Autodesk Fusion 360 part; units mm, degrees
sketch "Sketch1" plane through (0, 0, 0) normal (0, 0, 1) x (1, 0, 0) in component "Airfoil structure"
  spline S0 degree 5 poles (152.8506, 9.5306) (153.6754, 9.3537) (155.1958, 9.0287) (157.0885, 8.6275) (158.936, 8.2427) (160.6637, 7.8881) (162.4454, 7.5151) (164.8303, 6.998) (168.0437, 6.2836) (171.9513, 5.3996) (176.2204, 4.4167) (180.4193, 3.4264) (184.1364, 2.5129) (187.0894, 1.7283) (189.2467, 1.0645) (190.9412, 0.4268) (192.3181, -0.1665) (193.5665, -0.7111) (194.5238, -1.126) (195.0337, -1.3464) knots 0 0 0 0 0 0 0.066667 0.133333 0.2 0.266667 0.333333 0.4 0.466667 0.533333 0.6 0.666667 0.733333 0.8 0.866667 0.933333 1 1 1 1 1 1
  line L0 (148.4907, 10.4656) -> (157.2105, 8.5955)
  line L1 (191.9852, -0.0289) -> (198.0822, -2.6639)
  circle A0 centre (33.1388, 9.1296) radius 4.765
  circle A1 centre (116.1615, 7.0362) radius 3.175
  spline S1 degree 5 poles (-3.081, -1.3464) (-3.6016, -1.2536) (-4.5414, -1.0763) (-5.6463, -0.8353) (-6.5938, -0.5669) (-7.329, -0.2953) (-8.0513, 0.0089) (-9.0194, 0.5707) (-10.0683, 1.7874) (-10.9642, 3.2518) (-11.5103, 4.4866) (-11.5777, 5.0951) (-11.407, 5.643) (-11.0112, 6.6067) (-10.1307, 7.993) (-8.6022, 9.6431) (-6.4035, 11.272) (-4.1965, 12.5715) (-2.7349, 13.4061) (-1.8316, 13.8946) (-1.0216, 14.2664) (0.0955, 14.6934) (1.459, 15.1916) (2.6392, 15.6173) (3.2971, 15.8534) knots 0 0 0 0 0 0 0.05 0.1 0.15 0.2 0.25 0.3 0.35 0.4 0.45 0.5 0.55 0.6 0.65 0.7 0.75 0.8 0.85 0.9 0.95 1 1 1 1 1 1
  line L2 (0.5703, -1.9971) -> (-6.7323, -0.6957)
  line L3 (-0.0118, 14.6656) -> (6.606, 17.0412)
  line L4 (-8.4792, 9.8153) -> (-3.9569, 12.8132)
  line L5 (-11.5034, 4.2257) -> (-11.5345, 5.6935)
  line L6 (-7.2174, -0.5359) -> (-9.7443, 1.1286)
  spline S2 degree 5 poles (93.5688, 19.3646) (93.8188, 19.3387) (94.2829, 19.2905) (94.8714, 19.229) (95.4658, 19.1659) (96.0263, 19.1049) (96.567, 19.0445) (97.2368, 18.9678) (98.1315, 18.8622) (99.313, 18.7173) (100.8214, 18.5245) (102.3118, 18.3263) (103.5973, 18.1504) (104.53, 18.0207) (105.0153, 17.9528) knots 0 0 0 0 0 0 0.1 0.2 0.3 0.4 0.5 0.6 0.7 0.8 0.9 1 1 1 1 1 1
  line L7 (92.266, 19.4996) -> (94.8715, 19.2297)
  line L8 (103.6448, 18.1447) -> (106.3858, 17.761)
  spline S3 degree 5 poles (6.5765, 16.943) (6.9079, 17.0449) (7.5374, 17.2364) (8.3817, 17.4868) (9.3156, 17.7508) (10.2084, 17.9865) (10.8922, 18.156) (11.4504, 18.29) (11.9864, 18.4184) (12.6265, 18.5675) (13.504, 18.76) (14.4962, 18.9637) (15.447, 19.1503) (16.1786, 19.2906) (16.5688, 19.3646) knots 0 0 0 0 0 0 0.1 0.2 0.3 0.4 0.5 0.6 0.7 0.8 0.9 1 1 1 1 1 1
  line L9 (5.4107, 16.5846) -> (7.7424, 17.3015)
  line L10 (15.2328, 19.111) -> (17.9048, 19.6183)
  line L11 (152.4045, 9.626) -> (152.8506, 9.5306)
  line L12 (107.9851, 17.5282) -> (108.4359, 17.4637)
  line L13 (6.1441, 16.7993) -> (6.5765, 16.943)
  line L14 (128.8588, -1.3464) -> (132.3138, -1.3464)
  line L15 (149.471, 10.2539) -> (148.8431, 7.3203)
  line L16 (148.8431, 7.3203) -> (151.7767, 6.6925)
  line L17 (151.7767, 6.6925) -> (152.4045, 9.626)
  line L18 (3.2971, 15.8534) -> (4.243, 13.0064)
  line L19 (4.243, 13.0064) -> (7.09, 13.9524)
  line L20 (7.09, 13.9524) -> (6.1441, 16.7993)
  line L21 (160.8934, -1.3464) -> (160.8934, 1.6536)
  line L22 (160.8934, 1.6536) -> (163.8934, 1.6536)
  line L23 (163.8934, 1.6536) -> (163.8934, -1.3464)
  line L24 (132.3138, -1.3464) -> (160.8934, -1.3464)
  line L25 (163.8934, -1.3464) -> (195.0337, -1.3464)
  line L26 (3.4513, -1.3464) -> (3.4513, 1.6536)
  line L27 (3.4513, 1.6536) -> (6.4513, 1.6536)
  line L28 (6.4513, 1.6536) -> (6.4513, -1.3464)
  line L29 (-3.081, -1.3464) -> (3.4513, -1.3464)
  line L30 (105.0153, 17.9528) -> (107.9851, 17.5282)
  line L31 (19.5688, 19.3646) -> (19.5688, 16.3646)
  line L32 (19.5688, 16.3646) -> (16.5688, 16.3646)
  line L33 (16.5688, 16.3646) -> (16.5688, 19.3646)
  line L34 (90.5688, 19.3646) -> (90.5688, 16.3646)
  line L35 (90.5688, 16.3646) -> (93.5688, 16.3646)
  line L36 (93.5688, 16.3646) -> (93.5688, 19.3646)
  line L37 (113.7881, 13.5683) -> (110.8279, 14.0557)
  line L38 (110.8279, 14.0557) -> (111.3153, 17.0159)
  line L39 (113.7881, 13.5683) -> (114.2755, 16.5285)
  spline S4 degree 5 poles (108.4359, 17.4637) (108.6467, 17.433) (108.9931, 17.3831) (109.2865, 17.3426) (109.4547, 17.3194) (110.0313, 17.2264) (110.7239, 17.113) (111.2088, 17.0334) (111.3153, 17.0159) knots 0 0 0 0 0 0 0.066667 0.133333 0.2 0.217791 0.217791 0.217791 0.217791 0.217791 0.217791
  line L40 (107.9387, 17.5361) -> (108.933, 17.3913)
  line L41 (110.8712, 17.0888) -> (111.7595, 16.9429)
  spline S5 degree 5 poles (114.2755, 16.5285) (114.9096, 16.424) (116.2698, 16.2) (118.5862, 15.8186) (122.1455, 15.233) (126.9408, 14.4438) (131.5558, 13.6821) (135.521, 13.0215) (138.5596, 12.5011) (140.775, 12.0942) (142.7661, 11.6889) (144.7964, 11.2532) (146.8777, 10.807) (148.5577, 10.4484) (149.471, 10.2539) knots 0 0 0 0 0 0 0.1 0.2 0.3 0.4 0.5 0.6 0.7 0.8 0.9 1 1 1 1 1 1
  line L42 (111.4536, 16.9934) -> (117.0973, 16.0636)
  line L43 (143.5745, 11.5101) -> (155.3674, 8.9976)
  line L44 (56.6502, 19.3646) -> (56.6502, 16.3646)
  line L45 (56.6502, 16.3646) -> (53.6502, 16.3646)
  line L46 (53.6502, 16.3646) -> (53.6502, 19.3646)
  line L47 (19.5688, 19.3646) -> (53.6502, 19.3646)
  line L48 (56.6502, 19.3646) -> (90.5688, 19.3646)
  line L49 (68.1265, -1.3464) -> (68.1265, 1.6536)
  line L50 (68.1265, 1.6536) -> (65.1265, 1.6536)
  line L51 (65.1265, 1.6536) -> (65.1265, -1.3464)
  line L52 (6.4513, -1.3464) -> (65.1265, -1.3464)
  line L53 (68.1265, -1.3464) -> (128.8588, -1.3464)
  point P0 (-8.4808, 0.2964)
  point P1 (-11.5189, 4.9596)
  point P2 (-6.2181, 11.3142)
  point P3 (11.4183, 18.2822)
  point P4 (96.5722, 19.0435)
  point P5 (109.7229, 17.2753)
  point P6 (137.8507, 12.6179)
  point P7 (163.7248, 7.2358)
  point P8 (186.791, 1.7868)
  dimension "d38" = 77
  dimension "d53" = 9.53
  dimension "d54" = 6.35
  dimension "d59" = 3
  dimension "d67" = 3
extrude "Extrude2" add sketch "Sketch1" along normal blind 3 contours S0 L0 L1 S1 S2 L7 L8 S3 L11 L12 L13 L14 L15 L16 L17 L18 L19 L20 L21 L22 L23 L24 L25 L26 L27 L28 L29 L30 L31 L32 L33 L34 L35 L36 L37 L38 L39 S4 L40 L41 S5 L42 L44 L45 L46 L47 L48 L49 L50 L51 L52 L53
sketch "Sketch3" plane through (0, 0, 0) normal (0, 0, 1) x (1, 0, 0)
component "Airfoil structure" placed x (1, 0, 0) y (0, 1, 0) z (0, 0, 1) at (0, 0, 0)
Here's how the part is built. I have some questions about the finished solid (model axes, mm). Round coordinates to 2 decimals unless told otherwise and drop trailing zeros. Answer as CSV lines item,"result".
1. For pin 1 (5.5 mm diameter, centred on x = 116.16, y = 7.04, fed in from -Z); pin 2 (1.5 mm diameter, centred on y = 0.5, z = 1, fed in from -X); pin 3 (1.5 mm diameter, centred on y = -0.5, z = 1.5, fed in from +X); pin 4 (1.5 mm diameter, centred on x = 4.5, z = 1.5, fed in from -Y), each with a flat end and sliding along its axis, tell me the tip position at first contact or that it passes through.
Final values:
pin 1,"passes through"
pin 2,"stops at x = -9.55"
pin 3,"stops at x = 194.81"
pin 4,"stops at y = 1.65"
2. Thinking about a two-plate mould opening in X: for faces 1 (the face through (112.99, 6.9, 1.48)), 2 (the face through (67, 7, 3)), which applies, released by +X, released by -X, zero draft, split by the parting line, or undercut?
Final values:
face 1,"undercut"
face 2,"zero draft"
3. If I drill on L1, parallel to X at y = 9.75, z = 2.8; L2, parallel to Y at x = 33, z = 2.75; L3, parallel to Y at x = 36.5, z = 0.65, over which ranges is the centre line in solid material (lowest first)?
Final values:
L1,"x = -8.31 to 28.41, 37.86 to 114.51, 117.81 to 149.36"
L2,"y = -1.35 to 4.37, 13.89 to 19.36"
L3,"y = -1.35 to 5.75, 12.51 to 19.36"
4. If we section it at A-A on z = 2.4: Count the separate pieces of the cut face and the enclosed holes in it, plus the area to 3 significant figures.
Final values:
separate pieces,"1"
enclosed holes,"2"
area,"3,070 mm^2"
